from build123d import *

# Parameters (mm, degrees)
F0_R     = 35
F1_DEPTH = 375
F2_R     = 25
F3_DEPTH = 50
F4_R     = 25
F5_DEPTH = 50


with BuildPart() as f1:
    # F0 (on Right) → F1 (new body, symmetric)
    with BuildSketch(Plane.YZ):
        Circle(F0_R)
    extrude(amount=F1_DEPTH, both=True)

    # F2 (on face) → F3 (cut)
    with BuildSketch(Plane(origin=(-375, 0, 0), x_dir=(0, -1, 0), z_dir=(-1, 0, 0))):
        Circle(F2_R)
    extrude(amount=-F3_DEPTH, mode=Mode.SUBTRACT)

    # F4 (on face) → F5 (cut)
    with BuildSketch(Plane.YZ.offset(375)):
        Circle(F4_R)
    extrude(amount=-F5_DEPTH, mode=Mode.SUBTRACT)


solid = f1.part
Model file for the job. Use its own axes, mm. A direction names the side the tool comes from. Round coordinates to 2 decimals unless told otherwise and drop trailing zeros. Loops run counter-clockwise (first coordinate to the right, second up) from the corner with the lowest first, then second, coordinate; pieces in that order, holes last. Notation, with made-up numbers: (-30.75, 82.5) -> (-3.75, 82.5) arc R16 ccw to (-3.75, 87.5) -> close; hole circle Ø3 at (-8, 36). An arc over 180 degrees is marked (long way). Answer as CSV lines item,"result". Start each with the question number.
1) Tool access for faces 1 (the face through (325, 0, 0)), 2 (the face through (-325, 0, 0)), 3 (the face through (375, -24, 8)): list every direction of +Z, -Z, +X, -X, +Y, -Y with a clear straight run to the whole face (end or side of a thin tool).
2) Slice it at C-C (x = -28). List the corners of the cut face in (y, z), plus the area to 3 significant figures.
3) Slice it at A-A (z = 0). List the corners of the cut face in (x, y), plus the area to 3 significant figures.
4) Pin check, flat tips, straight feed: P1, Ø10, axis at x = 56, y = 15, coming from the -Z side; P2, Ø2, axis at x = -183, z = 27, coming from the +Y side; P3, Ø3, axis at y = -1.5, z = 7.5, coming from the -X side. Stop position of each tip, or through.
5) Mould opens along Y. For faces 4 (the face through (-375, -24, 8)), 5 (the face through (-350.35, -23.846, 7.509)), 6 (the face through (5, -28, -21)) say: +Y half, -Y half, draft (parallel to the pull), parting line (faces both ways), or undercut.
6) Probe line 1 along Z through (x, y) = (-344, 0); line 2 along X through (y, z) = (-24.5, 1.5); line 3 along Y through (x, z) = (-332.5, -4). List the from-to ranges inside material, lowest first.
Filled in:
1,face 1,"+X"
1,face 2,"-X"
1,face 3,"+Z, -Z, +X, +Y, -Y"
2,outline,"circle Ø70 at (0, 0)"
2,area,"3,850 mm2"
3,outline,"(-375, -35) -> (375, -35) -> (375, -25) -> (325, -25) -> (325, 25) -> (375, 25) -> (375, 35) -> (-375, 35) -> (-375, 25) -> (-325, 25) -> (-325, -25) -> (-375, -25) -> close"
3,area,"47,500 mm2"
4,P1,"stops at z = -33.54"
4,P2,"stops at y = 23.43"
4,P3,"stops at x = -325"
5,face 4,"draft"
5,face 5,"undercut"
5,face 6,"parting line"
6,line 1,"z = -35 to -25, 25 to 35"
6,line 2,"x = -325 to 325"
6,line 3,"y = -34.77 to -24.68, 24.68 to 34.77"
